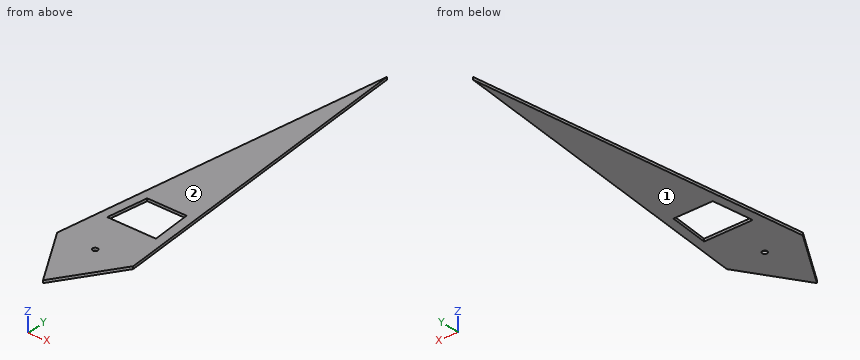
from build123d import *

# Parameters (mm, degrees)
SKETCH1_R           = 0.1
BOSS_EXTRUDE1_DEPTH = 0.1
CUT_EXTRUDE1_DEPTH  = 0.1


with BuildPart() as part:
    # Sketch1 → Boss-Extrude1 (new body)
    with BuildSketch(Plane.XY):
        Polygon((0, 13.302859744), (1.5, 0), (0, -2.380255614), (-1.5, 0), align=None)
        Circle(SKETCH1_R, mode=Mode.SUBTRACT)
    extrude(amount=BOSS_EXTRUDE1_DEPTH)

    # Sketch2 → Cut-Extrude1 (cut)
    with BuildSketch(Plane.XY.offset(0.1)):
        Polygon((-0.959190931, 1.658080162), (0.959190931, 1.658080162), (0.777629766, 3.268268638), (-0.777629766, 3.268268638), align=None)
    extrude(amount=-CUT_EXTRUDE1_DEPTH, mode=Mode.SUBTRACT)


solid = part.part
Build history of the part. All positions in model axes, mm. Face numbers are marked on the shaded views. Round coordinates to 2 decimals unless told otherwise and drop trailing zeros. Write each loop counter-clockwise with the first axis right and the second up, starting at its lowest first coordinate (ties: lowest second). Pieces come first, ordered by that corner, then holes. Notation, with made-up numbers: M -37,75.25 L -26,75.25 A32 cw -26,107.25 Z; hole C 23.25,-5 d8. An arc over 180 degrees is marked long. Answer as a JSON object with one key per item and string values. Group by question number.
(1) Flat gauge pin, fed straight in: pin 1 (1 mm diameter, centred on x = 0.5, y = 6.5, fed in from -Z). Where does the tip first touch, or does it go through?
(2) Mould opens along Z. For the marked faces 1 and 2 say: pulls with the +Z half, pulls with the -Z half, needs draft (parallel to the pull), parting line crosses it, or undercut.
(3) Cut at B-B (y = -0.25). Give the cut face in (x, z).
(4) Cut at A-A (x = -0.25). Give the cut face in (y, z).
(5) Cut at C-C (x = 1.25). Give the cut face in (y, z).
(6) Drill centre lines: L1, parallel to X at y = 0.75, z = 0.05; L2, parallel to X at y = 6.75, z = 0.05. Where is each one in solid material? Low to high.
Responses:
{
 "1": {"pin 1": "stops at z = 0"},
 "2": {"face 1": "pulls with the -Z half", "face 2": "pulls with the +Z half"},
 "3": {"outline": "M -1.34,0 L 1.34,0 L 1.34,0.1 L -1.34,0.1 Z"},
 "4": {"outline": "M -1.98,0 L 1.66,0 L 1.66,0.1 L -1.98,0.1 Z; M 3.27,0 L 11.09,0 L 11.09,0.1 L 3.27,0.1 Z"},
 "5": {"outline": "M -0.4,0 L 2.22,0 L 2.22,0.1 L -0.4,0.1 Z"},
 "6": {"L1": "x = -1.42 to 1.42", "L2": "x = -0.74 to 0.74"}
}
